Autodesk Inventor part; units mm, degrees
ref_plane "Work Plane1" through (29, 0, 0) normal (0, -1, 0) x (1, 0, 0)
ref_plane "YZ Plane" through (0, 0, 0) normal (1, 0, 0) x (0, 1, 0)
ref_plane "XZ Plane" through (0, 0, 0) normal (0, 1, 0) x (-1, 0, 0)
sketch "Sketch1" plane through (0, 0, 0) normal (0, 0, 1) x (1, 0, 0)
  line L0 (-0.6667, 0) -> (10, 0)
  line L1 (10, 0) -> (10, 1.5)
  line L2 (10, 1.5) -> (1.3067, 1.5)
  line L3 (1.3067, 1.5) -> (0.9999, 1.5)
  line L4 (0.9999, 1.5) -> (0, 1.5)
  line L5 (0, 1.5) -> (0, 2.75)
  line L6 (0, 2.75) -> (-3, 2.75)
  line L7 (-3, 2.75) -> (-3, 1.4434)
  line L8 (-3, 1.4434) -> (-1.5, 1.4434)
  line L9 (-1.5, 1.4434) -> (-0.6667, 0)
  line L10 (-5.6, 0) -> (12.6, 0)
  line L11 (0, -0.55) -> (0, 3.3)
  line L12 (1.3067, 1.5) -> (0, 1.5) construction
  dimension "d1" = 8.6933
  dimension "d2" = 0.3068
  dimension "d3" = 3
  dimension "d4" = 1.5
  dimension "d5" = 60
  dimension "d6" = 3
  dimension "d7" = 3
  dimension "d8" = 2.8868
  dimension "d9" = 5.5
  dimension "d26" = 10
revolve "Body" add sketch "Sketch1" angle 360 about axis through (-0.6667, 0, 0) along (1, 0, 0)
sketch "Sketch2" plane through (-3, 0, 0) normal (-1, 0, 0) x (0, 0, 1)
  circle A0 centre (0, 0) radius 1.4434
  line L0 (0, -3.85) -> (0, 3.85)
  line L1 (-3.85, 0) -> (3.85, 0)
  line L2 (1.4434, 0) -> (0.7217, -1.25)
  line L3 (0.7217, -1.25) -> (-0.7217, -1.25)
  line L4 (-0.7217, -1.25) -> (-1.4434, 0)
  line L5 (-1.4434, 0) -> (-0.7217, 1.25)
  line L6 (-0.7217, 1.25) -> (0.7217, 1.25)
  line L7 (0.7217, 1.25) -> (1.4434, 0)
  point P0 (0, 0)
extrude "Slot" add sketch "Sketch2" against normal up to next contours L7 A0 | A0 L2 | L6 L0 A0 | A0 L0 L3 | L0 L6 A0 | A0 L3 L0 | L4 A0 | A0 L5
fillet "Fillet1" radius 0.3 1 edges at (-3, -2.75, 0)
thread "Thread"
chamfer "Chamfer1" distance 0.3067 distance2 0.3067 1 edges at (10, -1.5, 0) measured on face at (10, -0.6587, -0.1791)
ref_plane "Work Plane1" through (29, 0, 0) normal (0, -1, 0) x (1, 0, 0)
fillet "Fillet2" radius 0.1 1 edges at (0, -1.5, 0)
equation "\"d1\" = GEL"
equation "\"d3\" = KOH"
equation "\"d4\" = INTI"
equation "\"d6\" = GD"
equation "\"d7\" = BDM"
equation "\"d8\" = 1.1547 * SW"
equation "\"d9\" = KOD"
equation "\"d26\" = NLG"
equation "\"d30\" = R"
equation "\"d17\" = RR"
equation "\"d13\" = GEL"
equation "\"d15\" = -0.5 * SPD + 0.5 * GD"
equation "\"d16\" = GUL"
equation "\"GD\" = NND"
equation "\"NLG\" = 10"
equation "\"GEL\" = 8.69327"
equation "\"KOD\" = 5.5"
equation "\"KOH\" = 3"
equation "\"INTI\" = 1.5"
equation "\"GAL\" = 0.61345 * PTC"
equation "\"GUL\" = 0.61345 * PTC"
equation "\"BDM\" = NND"
equation "\"SW\" = 2.5"
equation "\"RR\" = 0.3"
equation "\"SPD\" = 2.38655"
equation "\"R\" = 0.1"
equation "\"TOA\" = 30deg"
equation "\"THREADDIA\" = 3"
equation "\"PTC\" = 0.5"
equation "\"NND\" = 3"
equation "\"E0\" = 1.155 * SW"
equation "\"GD1\" = THREADDIA - 1.2269 * PTC"
properties part number "ANSI B18.3.1M - M3x0.5 x 10" material "Steel, Mild"
Part model, mm, in its own coordinate system. A direction names the side the tool comes from. Coordinates: 2 decimals unless noted, no trailing zeros. Loops run counter-clockwise (first coordinate to the right, second up) from the corner with the lowest first, then second, coordinate; pieces in that order, holes last. Notation, with made-up numbers: M 12.5,60 L 41.5,60 A34 cw 41.5,94 Z; hole C -22.5,46 d11. An arc over 180 degrees is marked long. Use a Markdown table: item, result. Add a question column.
Q1. Mould opens along Y. For faces 1 (the flat face through (-2.21, 0.63, 1.08)), 2 (the flat face through (-2, 1.25, 0)), 3 (the flat face through (10, 0, 0)), 4 (the cylindrical face through (4.83, -1.5, -0.07)) say: +Y half, -Y half, draft (parallel to the pull), parting line (faces both ways), or undercut.
Q2. Pin check, flat tips, straight feed: P1, Ø0.7, axis at x = -2, z = 0.5, coming from the -Y side; P2, Ø1.5, axis at x = -1, z = -2, coming from the +Y side. Stop position of each tip, or through.
Q3. Probe L1, parallel to Y at x = 9.75, z = 0; L2, parallel to X at y = -1.6, z = -0.65; L3, parallel to Z at x = -2, y = -0.7. List the from-to ranges inside material, lowest first.
Q4. Cut at B-B (x = -1). Write the cut outline in (y, z), and give its area (3 significant figures).
Q5. Which spindle directions (+Z, -Z, +X, -X, +Y, -Y) get a long thin tool onto all of the face, cutting with end or side? Do faces 5 (the flat face through (0, 2, 0)), 6 (the flat face through (-3, -1.1, 1.1)), 7 (the flat face through (-2.205, -0.616, 1.088)). Say none if no direction does.
Q6. Cut at A-A (x = 6). Write the cut outline in (y, z), and give its area (3 significant figures).
Worked out:
| question | item | result |
|---|---|---|
| 1 | face 1 | undercut |
| 1 | face 2 | undercut |
| 1 | face 3 | draft |
| 1 | face 4 | parting line |
| 2 | P1 | stops at y = -2.75 |
| 2 | P2 | stops at y = 2.45 |
| 3 | L1 | y = -1.44 to 1.44 |
| 3 | L2 | x = -3 to 0 |
| 3 | L3 | z = -2.66 to -1.04, 1.04 to 2.66 |
| 4 | outline | C 0,0 d5.5; hole C 0,0 d1.15 |
| 4 | area | 22.7 mm2 |
| 5 | face 5 | +X |
| 5 | face 6 | +Z, -Z, -X, +Y, -Y |
| 5 | face 7 | -X |
| 6 | outline | C 0,0 d3 |
| 6 | area | 7.07 mm2 |
